For this review, take the finished solid that the model builds, in its own axes (mm). Face numbers are marked on the shaded views. A direction names the side the tool comes from. Give positions to 0.01 mm unless a question says otherwise; leave off trailing zeros. Loops run counter-clockwise (first coordinate to the right, second up) from the corner with the lowest first, then second, coordinate; pieces in that order, holes last. Notation, with made-up numbers: (24.5, 85) -> (34.5, 85) arc R3 ccw to (34.5, 89) -> close; hole circle Ø7 at (20.25, 75.25). An arc over 180 degrees is marked (long way). Answer as CSV lines item,"result". Start each with the question number.
Item 1: Clearance check with flat-ended pins moving along their axes: P1, Ø5.5, axis at y = -13, z = 17, coming from the +X side; P2, Ø4, axis at x = 11, y = 8, coming from the +Z side; P3, Ø3.5, axis at y = 14.5, z = 23, coming from the -X side. State where each tip first meets the part, or that it passes through.
Item 2: Add section C-C on y = 19. State the section outline as (x, z) points.
Item 3: For L1, parallel to X at y = 19.5, z = 32.5; L2, parallel to Z at x = -12, y = -3; L3, parallel to Y at x = 11, z = 9.5, list the stretches that pass through material, from the lowest coordinate up. Write a range as from..to.
Item 4: Add section D-D on z = 5. State how many separate pieces and enclosed holes the cut face has, plus the area to 3 significant figures.
Item 5: Machinability: for the marked faces 5, 6 and 7, which of the approach directions +Z, -Z, +X, -X, +Y, -Y give a long, thin tool a straight path to every point of the face, cutting with its end or side? Answer none if there is none.
Item 6: Add section B-B on x = 0. State the section outline as (y, z) points, plus the area to 3 significant figures.
Item 7: The part is to be moulded in two halves that separate along X. For the marked faces 1, 2, 3 and 4, say which applies: +X half, -X half, draft (parallel to the pull), parting line (faces both ways), or undercut.
Item 8: Add section A-A on z = 40. State the section outline as (x, y) points.
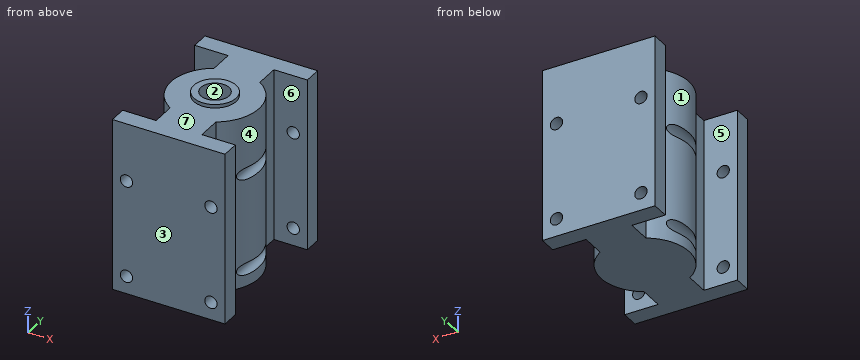
```python
from build123d import *

# Parameters (mm, degrees)
BOSS_EXTRUDE1_DEPTH = 49
SKETCH2_R           = 4
CUT_EXTRUDE1_DEPTH  = 47
SKETCH7_W           = 32
SKETCH7_H           = 5
BOSS_EXTRUDE2_DEPTH = 49
SKETCH8_R           = 1.75
CUT_EXTRUDE4_DEPTH  = 69.425141578
BOSS_EXTRUDE3_START = 1
SKETCH9_R           = 6
SKETCH9_R_2         = 4
BOSS_EXTRUDE3_DEPTH = 1


with BuildPart() as part:
    # Sketch1 → Boss-Extrude1 (new body)
    with BuildSketch(Plane.XY):
        with BuildLine():
            Line((-6.5, 17.5), (6.5, 17.5))
            Line((6.5, 17.5), (6.5, 10.677078252))
            ThreePointArc((6.5, 10.677078252), (12.5, 0), (6.5, -10.677078252))
            Line((6.5, -10.677078252), (6.5, -17.5))
            Line((6.5, -17.5), (-6.5, -17.5))
            Line((-6.5, -17.5), (-6.5, -10.677078252))
            ThreePointArc((-6.5, -10.677078252), (-12.5, 0), (-6.5, 10.677078252))
            Line((-6.5, 10.677078252), (-6.5, 17.5))
        make_face()
    extrude(amount=BOSS_EXTRUDE1_DEPTH)

    # Sketch2 → Cut-Extrude1 (cut)
    with BuildSketch(Plane.XY.offset(49)):
        Circle(SKETCH2_R)
    extrude(amount=-CUT_EXTRUDE1_DEPTH, mode=Mode.SUBTRACT)

    # Sketch7 → Boss-Extrude2 (add)
    with BuildSketch(Plane.XY):
        with Locations((0, 20)):
            Rectangle(SKETCH7_W, SKETCH7_H)
        with Locations((0, -20)):
            Rectangle(SKETCH7_W, SKETCH7_H)
    extrude(amount=BOSS_EXTRUDE2_DEPTH)

    # Sketch8 → Cut-Extrude4 (cut, through all)
    with BuildSketch(Plane(origin=(0, 22.5, 0), x_dir=(1, 0, 0), z_dir=(0, 1, 0))):
        with Locations(Location((-12, -5, 0), (0, 0, 270))):
            Circle(SKETCH8_R)
        with Locations(Location((-12, -32.5, 0), (0, 0, 270))):
            Circle(SKETCH8_R)
        with Locations(Location((12, -32.5, 0), (0, 0, 270))):
            Circle(SKETCH8_R)
        with Locations(Location((12, -5, 0), (0, 0, 270))):
            Circle(SKETCH8_R)
    extrude(amount=-CUT_EXTRUDE4_DEPTH, mode=Mode.SUBTRACT)

    # Sketch9 → Boss-Extrude3 (add)
    with BuildSketch(Plane.XY.offset(49).offset(BOSS_EXTRUDE3_START)):
        Circle(SKETCH9_R)
        Circle(SKETCH9_R_2, mode=Mode.SUBTRACT)
    extrude(amount=-BOSS_EXTRUDE3_DEPTH)


solid = part.part
```
Computed values:
1,P1,"x = 7.15"
1,P2,"z = 49"
1,P3,"x = -6.5"
2,outline,"(-16, 0) -> (16, 0) -> (16, 49) -> (-16, 49) -> close; hole circle Ø3.5 at (-12, 5); hole circle Ø3.5 at (-12, 32.5); hole circle Ø3.5 at (12, 5); hole circle Ø3.5 at (12, 32.5)"
3,L1,"-16..-13.75, -10.25..10.25, 13.75..16"
3,L2,"0..3.25, 6.75..30.75, 34.25..49"
3,L3,"-22.5..-17.5, -5.94..5.94, 17.5..22.5"
4,separate pieces,"5"
4,enclosed holes,"1"
4,area,"792 mm²"
5,face 5,"+Z, -Z, -X"
5,face 6,"+Z, -Z, +X"
5,face 7,"+Z"
6,outline,"(-22.5, 0) -> (22.5, 0) -> (22.5, 49) -> (6, 49) -> (6, 50) -> (4, 50) -> (4, 2) -> (-4, 2) -> (-4, 50) -> (-6, 50) -> (-6, 49) -> (-22.5, 49) -> close"
6,area,"1,830 mm²"
7,face 1,"-X half"
7,face 2,"undercut"
7,face 3,"draft"
7,face 4,"+X half"
8,outline,"(-16, -22.5) -> (16, -22.5) -> (16, -17.5) -> (6.5, -17.5) -> (6.5, -10.68) arc R12.5 ccw to (6.5, 10.68) -> (6.5, 17.5) -> (16, 17.5) -> (16, 22.5) -> (-16, 22.5) -> (-16, 17.5) -> (-6.5, 17.5) -> (-6.5, 10.68) arc R12.5 ccw to (-6.5, -10.68) -> (-6.5, -17.5) -> (-16, -17.5) -> close; hole circle Ø8 at (0, 0)"
